CAD build for the part. Positions are in the model's coordinates, mm. Face numbers are marked on the shaded views. A direction names the side the tool comes from. Coordinates: 2 decimals unless noted, no trailing zeros. Write each loop counter-clockwise with the first axis right and the second up, starting at its lowest first coordinate (ties: lowest second). Pieces come first, ordered by that corner, then holes. Notation, with made-up numbers: (-24.5, 37) -> (-1.5, 37) arc R28 cw to (-1.5, 58) -> close; hole circle Ø5 at (80.5, 3). An arc over 180 degrees is marked (long way). Answer as CSV lines item,"result". Start each with the question number.
```python
from build123d import *

# Parameters (mm, degrees)
SKETCH1_W           = 381
SKETCH1_H           = 457.2
SKETCH1_W_2         = 366
SKETCH1_H_2         = 442.1
BOSS_EXTRUDE1_DEPTH = 120
SKETCH2_W           = 366
SKETCH2_H           = 442.1
BOSS_EXTRUDE2_DEPTH = 10
FILLET1_R           = 20
CUT_EXTRUDE1_DEPTH  = 10


with BuildPart() as part:
    # Sketch1 → Boss-Extrude1 (new body)
    with BuildSketch(Plane(origin=(0, 0, 0), x_dir=(1, 0, 0), z_dir=(0, 1, 0))):
        with Locations((190.5, 228.6)):
            Rectangle(SKETCH1_W, SKETCH1_H)
        with Locations((190.5, 228.65)):
            Rectangle(SKETCH1_W_2, SKETCH1_H_2, mode=Mode.SUBTRACT)
    extrude(amount=BOSS_EXTRUDE1_DEPTH)

    # Sketch2 → Boss-Extrude2 (add)
    with BuildSketch(Plane.XZ):
        with Locations((190.5, -228.65)):
            Rectangle(SKETCH2_W, SKETCH2_H)
    extrude(amount=-BOSS_EXTRUDE2_DEPTH)

    # Fillet1
    fillet1_edges = [part.edges().sort_by_distance(p)[0] for p in [
        (0, 60, -457.2),
        (381, 60, 0),
        (0, 60, 0),
    ]]
    fillet(fillet1_edges, radius=FILLET1_R)

    # Sketch3 → Cut-Extrude1 (cut)
    with BuildSketch(Plane(origin=(381, 0, 0), x_dir=(0, 0, -1), z_dir=(1, 0, 0))):
        with BuildLine():
            Line((399.7, 87.25), (399.7, 90))
            Line((399.7, 90), (402.45, 90))
            ThreePointArc((402.45, 90), (397.755456352, 91.944543648), (399.7, 87.25))
        make_face()
        with BuildLine():
            Line((402.45, 90), (399.7, 90))
            Line((399.7, 90), (399.7, 87.25))
            ThreePointArc((399.7, 87.25), (401.644543648, 88.055456352), (402.45, 90))
        make_face()
        with BuildLine():
            ThreePointArc((452.45, 90), (449.7, 92.75), (446.95, 90))
            Line((446.95, 90), (449.7, 90))
            Line((449.7, 90), (449.7, 87.25))
            ThreePointArc((449.7, 87.25), (451.644543648, 88.055456352), (452.45, 90))
        make_face()
        with BuildLine():
            Line((449.7, 90), (446.95, 90))
            ThreePointArc((446.95, 90), (447.755456352, 88.055456352), (449.7, 87.25))
            Line((449.7, 87.25), (449.7, 90))
        make_face()
        with BuildLine():
            ThreePointArc((452.45, 30), (451.644543648, 31.944543648), (449.7, 32.75))
            Line((449.7, 32.75), (449.7, 30))
            Line((449.7, 30), (446.95, 30))
            ThreePointArc((446.95, 30), (449.7, 27.25), (452.45, 30))
        make_face()
        with BuildLine():
            Line((449.7, 30), (449.7, 32.75))
            ThreePointArc((449.7, 32.75), (447.755456352, 31.944543648), (446.95, 30))
            Line((446.95, 30), (449.7, 30))
        make_face()
        with BuildLine():
            ThreePointArc((402.45, 30), (401.644543648, 31.944543648), (399.7, 32.75))
            Line((399.7, 32.75), (399.7, 30))
            Line((399.7, 30), (402.45, 30))
        make_face()
        with BuildLine():
            Line((399.7, 30), (399.7, 32.75))
            ThreePointArc((399.7, 32.75), (397.755456352, 28.055456352), (402.45, 30))
            Line((402.45, 30), (399.7, 30))
        make_face()
    extrude(amount=-CUT_EXTRUDE1_DEPTH, mode=Mode.SUBTRACT)


solid = part.part
```
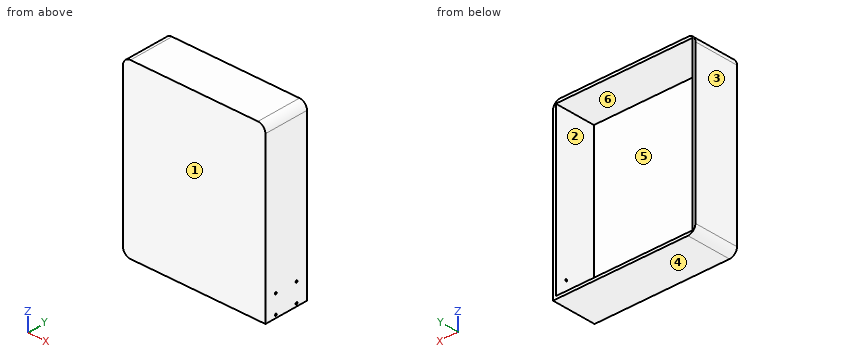
1. Cut at B-B (x = 313). Give the cut face in (y, z), then the cut area to 3 significant figures.
2. Wall check: line 1 (Y direction, x = 379, z = -399); line 2 (X direction, y = 68.5, z = -394); line 3 (Z direction, x = 133, y = 64). Give the ranges that are in metal, low to high.
3. Cut at C-C (z = -198). Give the cut face in (x, y).
4. Cut at A-A (y = 57). Give the cut face in (x, z), then the cut area to 3 significant figures.
5. Mould opens along Z. For the marked faces 3, 4, 5 and 6 say: pulls with the +Z half, pulls with the -Z half, needs draft (parallel to the pull), parting line crosses it, or undercut.
6. Tool access for the marked faces 1 and 2: list every direction of +Z, -Z, +X, -X, +Y, -Y with a clear straight run to the whole face (end or side of a thin tool).
7. Flat gauge pins, fed straight in: P1, Ø2, axis at x = 79, z = -137.5, coming from the +Y side; P2, Ø0.8, axis at y = 90, z = -451, coming from the +X side; P3, Ø8, axis at x = 233.5, z = -125, coming from the -Y side. Where does each tip first touch, or does it go through?
Geometry check:
1,outline,"(0, -457.2) -> (120, -457.2) -> (120, -449.7) -> (10, -449.7) -> (10, -7.6) -> (120, -7.6) -> (120, 0) -> (0, 0) -> close"
1,area,"6,230 mm²"
2,line 1,"0 to 27.34, 32.66 to 87.34, 92.66 to 120"
2,line 2,"0 to 7.5, 373.5 to 381"
2,line 3,"-457.2 to -449.7, -7.6 to 0"
3,outline,"(0, 0) -> (381, 0) -> (381, 120) -> (373.5, 120) -> (373.5, 10) -> (7.5, 10) -> (7.5, 120) -> (0, 120) -> close"
4,outline,"(0, -437.2) arc R20 ccw to (20, -457.2) -> (381, -457.2) -> (381, -20) arc R20 ccw to (361, 0) -> (20, 0) arc R20 ccw to (0, -20) -> close; hole (7.5, -449.7) -> (373.5, -449.7) -> (373.5, -7.6) -> (7.5, -7.6) -> close"
4,area,"12,100 mm²"
5,face 3,"needs draft"
5,face 4,"pulls with the -Z half"
5,face 5,"undercut"
5,face 6,"undercut"
6,face 1,"+Z, -Z, +X, -X, -Y"
6,face 2,"+Y"
7,P1,"y = 10"
7,P2,"x = 371"
7,P3,"y = 0"
